from build123d import *

# Parameters (mm, degrees)
F0_R     = 1.75
F2_DEPTH = 2
F1_W     = 4.5
F1_H     = 1.6
F1_W_2   = 2.5
F1_H_2   = 6.1
F1_R     = 6.5
F3_DEPTH = 2.001
F4_R     = 3


with BuildPart() as f2:
    # F0 (on Top) → F2 (new body)
    with BuildSketch(Plane.XY):
        Polygon((38.288459, 48.664646), (-37.211541, 48.664646), (-37.211541, -40.835354), (3.788459, -40.835354), (38.288459, -1.335354), align=None)
        with Locations((-32.461541, -36.085354)):
            Circle(F0_R, mode=Mode.SUBTRACT)
        with Locations((33.538459, 3.414646)):
            Circle(F0_R, mode=Mode.SUBTRACT)
        with Locations((-32.461541, 43.914646)):
            Circle(F0_R, mode=Mode.SUBTRACT)
        with Locations((33.538459, 43.914646)):
            Circle(F0_R, mode=Mode.SUBTRACT)
    extrude(amount=F2_DEPTH)

    # F1 (on Top) → F3 (cut, through all)
    with BuildSketch(Plane.XY):
        Polygon((-12.211541, 7.114646), (-12.211541, 9.314646), (-15.211541, 9.314646), (-19.711541, 9.314646), (-22.711541, 9.314646), (-22.711541, 7.114646), (-22.711541, 1.014646), (-22.711541, -1.185354), (-12.211541, -1.185354), (-12.211541, 1.014646), align=None)
        with Locations((-17.461541, 10.114646)):
            Rectangle(F1_W, F1_H)
        with Locations((-10.961541, 4.064646)):
            Rectangle(F1_W_2, F1_H_2)
        with Locations((-23.961541, 4.064646)):
            Rectangle(F1_W_2, F1_H_2)
        Polygon((14.788459, 32.864646), (14.788459, 35.064646), (11.788459, 35.064646), (7.288459, 35.064646), (4.288459, 35.064646), (4.288459, 32.864646), (4.288459, 26.764646), (4.288459, 24.564646), (14.788459, 24.564646), (14.788459, 26.764646), align=None)
        with Locations((9.538459, 35.864646)):
            Rectangle(F1_W, F1_H)
        with Locations((16.038459, 29.814646)):
            Rectangle(F1_W_2, F1_H_2)
        with Locations((3.038459, 29.814646)):
            Rectangle(F1_W_2, F1_H_2)
        Polygon((-12.211541, -14.985354), (-12.211541, -12.785354), (-15.211541, -12.785354), (-19.711541, -12.785354), (-22.711541, -12.785354), (-22.711541, -14.985354), (-22.711541, -21.085354), (-22.711541, -23.285354), (-12.211541, -23.285354), (-12.211541, -21.085354), align=None)
        with Locations((-17.461541, -11.985354)):
            Rectangle(F1_W, F1_H)
        with Locations((-10.961541, -18.035354)):
            Rectangle(F1_W_2, F1_H_2)
        with Locations((-23.961541, -18.035354)):
            Rectangle(F1_W_2, F1_H_2)
        with Locations((-17.461541, 30.164646)):
            Circle(F1_R)
    extrude(amount=F3_DEPTH, mode=Mode.SUBTRACT)

    # F4
    f4_edges = [f2.edges().sort_by_distance(p)[0] for p in [
        (-37.211541, 48.664646, 1),
        (38.288459, 48.664646, 1),
        (38.288459, -1.335354, 1),
        (3.788459, -40.835354, 1),
        (-37.211541, -40.835354, 1),
    ]]
    fillet(f4_edges, radius=F4_R)


solid = f2.part
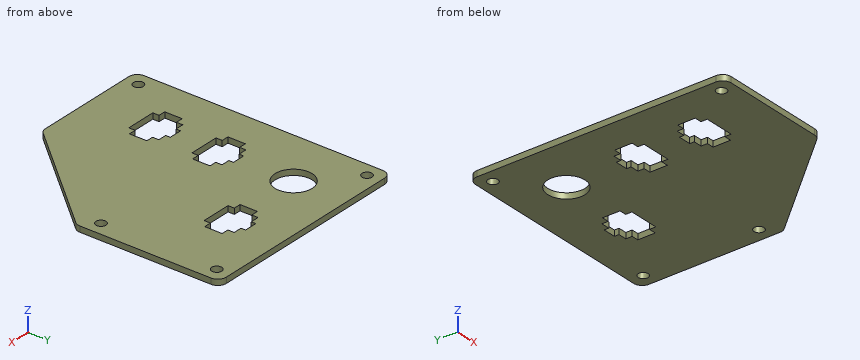
Could you check a few things on this model? Use its own coordinates, in mm. Give positions to 0.01 mm unless a question says otherwise; leave off trailing zeros. Order: outer loops, then holes, each group sorted by start corner. A loop starts at its lowest first (then second) coordinate and runs counter-clockwise, first axis right, second up.
Item 1: If we section it at C-C, the plane z = 0.5: Count the separate pieces of the cut face and the enclosed holes in it, plus the area to 3 significant figures.
Item 2: I need wall thicknesses on line 1 (Y direction, x = 33, z = 1.1); line 2 (X direction, y = 29.5, z = 0.4); line 3 (X direction, y = 26.5, z = 0.65). Which ranges of each line are inside material? Lowest first, please.
Item 3: If we section it at A-A, the plane x = -16.5: Write out the boundary of the cut face in (y, z).
Item 4: If we section it at D-D, the plane y = -25: Write out the boundary of the cut face in (x, z).
Item 5: If we section it at B-B, the plane x = 13.5: Write out the boundary of the cut face in (y, z), plus the area to 3 significant figures.
Values:
1. separate pieces: 1
1. enclosed holes: 8
1. area: 5,450 mm2
2. line 1: y = -7.39 to 1.75, 5.08 to 42.25, 45.58 to 48.66
2. line 2: x = -37.21 to -23.93, -11 to 1.79, 17.29 to 38.29
2. line 3: x = -37.21 to -22.83, -12.09 to 4.29, 14.79 to 38.29
3. outline: (-40.84, 0) - (-23.29, 0) - (-23.29, 2) - (-40.84, 2) - close; (-11.19, 0) - (-1.19, 0) - (-1.19, 2) - (-11.19, 2) - close; (10.91, 0) - (23.74, 0) - (23.74, 2) - (10.91, 2) - close; (36.59, 0) - (48.66, 0) - (48.66, 2) - (36.59, 2) - close
4. outline: (-37.21, 0) - (17.62, 0) - (17.62, 2) - (-37.21, 2) - close
5. outline: (-29.72, 0) - (24.56, 0) - (24.56, 2) - (-29.72, 2) - close; (35.06, 0) - (48.66, 0) - (48.66, 2) - (35.06, 2) - close
5. area: 136 mm2
